Work out the finished part from the listing and answer in its coordinate system (mm). Face numbers are marked on the shaded views. Round coordinates to 2 decimals unless told otherwise and drop trailing zeros. Write each loop counter-clockwise with the first axis right and the second up, starting at its lowest first coordinate (ties: lowest second). Pieces come first, ordered by that corner, then holes.
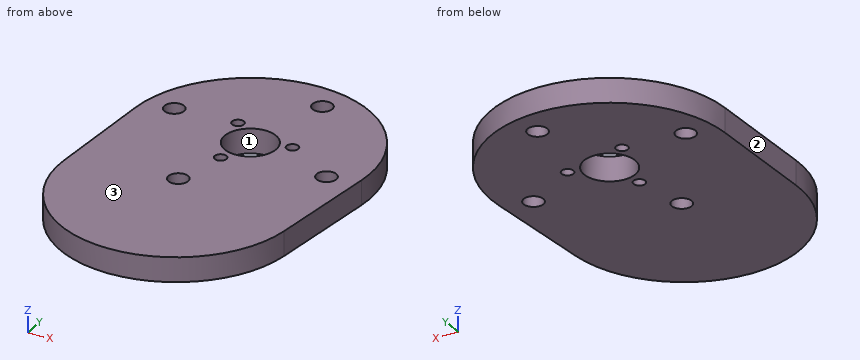
from build123d import *

# Parameters (mm, degrees)
SKETCH1_R           = 2.5
SKETCH1_R_2         = 6.5
BOSS_EXTRUDE1_DEPTH = 6.2
CUT_EXTRUDE1_REACH  = 68.667
SKETCH2_R           = 1.5


with BuildPart() as part:
    # Sketch1 → Boss-Extrude1 (new body)
    with BuildSketch(Plane.XY):
        with BuildLine():
            Line((25.948954725, -32.665145778), (29.742076772, -3.925413261))
            ThreePointArc((29.742076772, -3.925413261), (3.103448276, 29.839045038), (-29.913301505, 2.279121121))
            Line((-29.913301505, 2.279121121), (-32.115613465, -26.626065646))
            ThreePointArc((-32.115613465, -26.626065646), (-6.020689655, -57.887747374), (25.948954725, -32.665145778))
        make_face()
        with Locations(Location((22.196999252, -6.024385794, 0), (0, 0, 180))):
            Circle(SKETCH1_R, mode=Mode.SUBTRACT)
        with Locations(Location((-22.196999252, 6.024385794, 0), (0, 0, 180))):
            Circle(SKETCH1_R, mode=Mode.SUBTRACT)
        with Locations(Location((6.024385794, 22.196999252, 0), (0, 0, 180))):
            Circle(SKETCH1_R, mode=Mode.SUBTRACT)
        with Locations(Location((-6.024385794, -22.196999252, 0), (0, 0, 180))):
            Circle(SKETCH1_R, mode=Mode.SUBTRACT)
        with Locations(Location((0, 0, 0), (0, 0, 180))):
            Circle(SKETCH1_R_2, mode=Mode.SUBTRACT)
    extrude(amount=BOSS_EXTRUDE1_DEPTH)

    # Sketch2 → Cut-Extrude1 (cut, up to next)
    with BuildSketch(Plane.XY.offset(6.2), mode=Mode.PRIVATE) as cut_extrude1_sk1:
        with Locations((9.184169665, 2.42920307)):
            Circle(SKETCH2_R)
    cut_extrude1_tool1 = extrude(cut_extrude1_sk1.sketch, amount=-CUT_EXTRUDE1_REACH, mode=Mode.PRIVATE) & part.part
    # Sketch2 → Cut-Extrude1 (cut, up to next)
    with BuildSketch(Plane.XY.offset(6.2), mode=Mode.PRIVATE) as cut_extrude1_sk2:
        with Locations((-6.695836403, 6.739122708)):
            Circle(SKETCH2_R)
    cut_extrude1_tool2 = extrude(cut_extrude1_sk2.sketch, amount=-CUT_EXTRUDE1_REACH, mode=Mode.PRIVATE) & part.part
    # Sketch2 → Cut-Extrude1 (cut, up to next)
    with BuildSketch(Plane.XY.offset(6.2), mode=Mode.PRIVATE) as cut_extrude1_sk3:
        with Locations((-2.488333263, -9.168325778)):
            Circle(SKETCH2_R)
    cut_extrude1_tool3 = extrude(cut_extrude1_sk3.sketch, amount=-CUT_EXTRUDE1_REACH, mode=Mode.PRIVATE) & part.part
    add(cut_extrude1_tool1.solids().sort_by_distance((9.18417, 2.429203, 6.2))[0], mode=Mode.SUBTRACT)
    add(cut_extrude1_tool2.solids().sort_by_distance((-6.695836, 6.739123, 6.2))[0], mode=Mode.SUBTRACT)
    add(cut_extrude1_tool3.solids().sort_by_distance((-2.488333, -9.168326, 6.2))[0], mode=Mode.SUBTRACT)


solid = part.part
Q1. Given pin 1 (2.5 mm diameter, centred on x = -2.49, y = -9.17, fed in from -Z); pin 2 (3 mm diameter, centred on y = -8.5, z = 4.5, fed in from -X), each flat-ended and moving along its own axis, determine where each tip first touches the part or whether it passes through.
Q2. Find the intervals of material crossed by L1, parallel to X at y = 7.5, z = 4; L2, parallel to X at y = 3, z = 2; L3, parallel to Y at x = 1, z = 3.75, in increasing order.
Q3. The mould has two halves that part along Y. Classify the marked faces 1, 2 and 3: +Y half, -Y half, draft (parallel to the pull), parting line (faces both ways), or undercut.
Q4. Find section D-D (x = -27.5). Determine the outline of the cut face in (y, z), plus the area to 3 significant figures.
Q5. Find section A-A (y = 0). Determine the outline of the cut face in (x, z).
Q6. Find section C-C (x = 0). Determine the outline of the cut face in (y, z).
Q7. Find section B-B (z = 2.25). Count the separate pieces of the cut face and the enclosed holes in it, plus the area to 3 significant figures.
Report:
1. pin 1: passes through
1. pin 2: stops at x = -30.85
2. L1: x = -29.05 to -24.22, -20.18 to -7.99, -5.4 to 29.05
2. L2: x = -29.85 to -5.77, 5.77 to 7.8, 10.57 to 29.85
2. L3: y = -57.77 to -6.42, 6.42 to 29.98
3. face 1: undercut
3. face 2: +Y half
3. face 3: draft
4. outline: (-44.73, 0) - (11.99, 0) - (11.99, 6.2) - (-44.73, 6.2) - close
4. area: 352 mm2
5. outline: (-30.09, 0) - (-6.5, 0) - (-6.5, 6.2) - (-30.09, 6.2) - close; (6.5, 0) - (30, 0) - (30, 6.2) - (6.5, 6.2) - close
6. outline: (-57.89, 0) - (-6.5, 0) - (-6.5, 6.2) - (-57.89, 6.2) - close; (6.5, 0) - (30, 0) - (30, 6.2) - (6.5, 6.2) - close
7. separate pieces: 1
7. enclosed holes: 8
7. area: 4,240 mm2
